Verification items for the finished model (mm, model axes). A direction names the side the tool comes from. Round coordinates to 2 decimals unless told otherwise and drop trailing zeros. Write each loop counter-clockwise with the first axis right and the second up, starting at its lowest first coordinate (ties: lowest second). Pieces come first, ordered by that corner, then holes. Notation, with made-up numbers: M -7,-38.75 L 40,-38.75 A15 cw 40,-28.75 Z; hole C 27.25,31 d7. An arc over 180 degrees is marked long. One line per question, with ' | ' between items. Start each with the question number.
Q1. Cross-section at A-A (y = 14.5). Record the boundary of the cut face in (x, z).
Q2. Cross-section at D-D (x = -20.5). Record the boundary of the cut face in (y, z), then the cut area to 3 significant figures.
Q3. Release check for a two-part mould opening along X. For faces 1 (the face through (33, 0, 1)), 2 (the face through (-5.93, 37.42, 1.48)), 3 (the face through (-0.02, 42.73, 1.52)) record: released by +X, released by -X, zero draft, split by the parting line, or undercut.
Q4. Tool access check on faces 4 (the face through (-27, 33, 1)), 5 (the face through (12.275, 33.815, 1.521)), 6 (the face through (27, 33, 1)). Record the directions out of +Z, -Z, +X, -X, +Y, -Y that give a thin tool (end or side, any length) a straight path to the whole face; none if there is none.
Q5. Gauge pin test, flat ends, axial feed: pin 1 (1.5 mm diameter, centred on x = -28, z = 1.5, fed in from +Y); pin 2 (5 mm diameter, centred on x = 1.5, y = 29.5, fed in from -Z). Record the tip position at first contact, or that the pin passes through.
Q6. Thickness scan on line 1 along X through (y, z) = (10, 2.4); line 2 along Y through (x, z) = (11, 0.9); line 3 along Y through (x, z) = (5.5, 0.6). Record the ranges inside material, lowest first. Write a range as from..to.
Q7. Cross-section at C-C (x = 3.5). Record the boundary of the cut face in (y, z).
Q8. Cross-section at B-B (z = 0.95). Record the boundary of the cut face in (x, y), then the cut area to 3 significant figures.
from build123d import *

# Parameters (mm, degrees)
SKETCH1_W           = 56
SKETCH1_H           = 56
BOSS_EXTRUDE1_DEPTH = 3
FILLET1_R           = 3
FILLET2_R           = 1


with BuildPart() as part:
    # Sketch1 → Boss-Extrude1 (new body)
    with BuildSketch(Plane.XY):
        Polygon((-23, 33), (0, 43), (23, 33), (33, 33), (33, -33), (-33, -33), (-33, 33), align=None)
        Rectangle(SKETCH1_W, SKETCH1_H, mode=Mode.SUBTRACT)
        Polygon((-16.1, 33), (0, 40), (16.1, 33), align=None, mode=Mode.SUBTRACT)
    extrude(amount=BOSS_EXTRUDE1_DEPTH)

    # Fillet1
    fillet1_edges = [part.edges().sort_by_distance(p)[0] for p in [
        (33, -33, 1.5),
        (-33, -33, 1.5),
        (-33, 33, 1.5),
        (-23, 33, 1.5),
        (0, 43, 1.5),
        (23, 33, 1.5),
        (33, 33, 1.5),
        (28, -28, 1.5),
        (28, 28, 1.5),
        (-28, 28, 1.5),
        (-28, -28, 1.5),
    ]]
    fillet(fillet1_edges, radius=FILLET1_R)

    # Fillet2
    fillet2_edges = [part.edges().sort_by_distance(p)[0] for p in [
        (-16.1, 33, 1.5),
        (16.1, 33, 1.5),
    ]]
    fillet(fillet2_edges, radius=FILLET2_R)


solid = part.part
Determined:
1) outline: M -33,0 L -28,0 L -28,3 L -33,3 Z; M 28,0 L 33,0 L 33,3 L 28,3 Z
2) outline: M -33,0 L -28,0 L -28,3 L -33,3 Z; M 28,0 L 34.09,0 L 34.09,3 L 28,3 Z | area: 33.3 mm²
3) face 1: released by +X | face 2: undercut | face 3: split by the parting line
4) face 4: +Z, -Z, -X, +Y | face 5: +Z, -Z | face 6: +Z, -Z, +X, +Y
5) pin 1: stops at y = 33 | pin 2: stops at z = 0
6) line 1: x = -33..-28, 28..33 | line 2: y = -33..-28, 28..33, 35.22..38.22 | line 3: y = -33..-28, 28..33, 37.61..40.61
7) outline: M -33,0 L -28,0 L -28,3 L -33,3 Z; M 28,0 L 33,0 L 33,3 L 28,3 Z; M 38.48,0 L 41.48,0 L 41.48,3 L 38.48,3 Z
8) outline: M -33,-30 A3 ccw -30,-33 L 30,-33 A3 ccw 33,-30 L 33,30 A3 ccw 30,33 L 23.62,33 A3 cw 22.43,33.25 L 1.2,42.48 A3 ccw -1.2,42.48 L -22.43,33.25 A3 cw -23.62,33 L -30,33 A3 ccw -33,30 Z; hole M -28,-25 A3 ccw -25,-28 L 25,-28 A3 ccw 28,-25 L 28,25 A3 ccw 25,28 L -25,28 A3 ccw -28,25 Z; hole M -11.69,34.92 A1 ccw -11.29,33 L 11.29,33 A1 ccw 11.69,34.92 L 0,40 Z | area: 1,340 mm²
